For this review, take the finished solid that the model builds, in its own axes (mm). A direction names the side the tool comes from. Coordinates: 2 decimals unless noted, no trailing zeros. Write each loop counter-clockwise with the first axis right and the second up, starting at its lowest first coordinate (ties: lowest second). Pieces come first, ordered by that corner, then holes.
1) We need section A-A on x = 8.5. Write out the cut boundary in (y, z), then the cut area to 3 significant figures.
2) Insertion check: P1, Ø4, axis at y = 173, z = 5, coming from the -X side; P2, Ø20, axis at y = 129.5, z = 21, coming from the -X side; P3, Ø8, axis at x = -132.5, y = 162.5, coming from the -Z side. Each pin has a flat end and moves straight along its axis. Give the tip position at first contact, or say it passes through.
3) To check wall thickness, follow line 1 along X through (y, z) = (119, 62); line 2 along X through (y, z) = (77, -11); line 3 along Z through (x, y) = (95.5, 18). State the ranges of each line that lie inside material, in increasing order.
4) For faces 1 (the face through (30, 121, 35)), 2 (the face through (-30, 121, 35)), 3 (the face through (0.42, 150.516, 39.308)), 4 (the face through (225.952, 56.186, -8.941)), 5 (the face through (0.42, 91.14, 30.64)), list the 3-axis set-ups (+Z, -Z, +X, -X, +Y, -Y) from which the entire face can be reached by the end or side of a thin tool; tool diameter is ignored.
5) Mouldability with a two-part tool opening along X and no side actions: class faces 6 (the face through (-137.606, 96.84, -3.634)), 7 (the face through (-226.16, 56.69, -8.94)), 8 (the face through (-2, 0, -17)) as pulls with the +X half, pulls with the -X half, needs draft (parallel to the pull), parting line crosses it, or undercut.
from build123d import *

# Parameters (mm, degrees)
BOSS_EXTRUDE1_START     = -25
BOSS_EXTRUDE1_DEPTH     = 50
CUT_EXTRUDE1_DEPTH      = 341.53226913
CUT_EXTRUDE1_DEPTH_BACK = 341.53226913
BOSS_EXTRUDE3_DEPTH     = 30
CUT_EXTRUDE2_DEPTH      = 350.338594582
CUT_EXTRUDE2_DEPTH_BACK = 350.338594582
SKETCH4_R               = 20
CUT_EXTRUDE3_DEPTH      = 350.338594582
CUT_EXTRUDE3_DEPTH_BACK = 350.338594582
SKETCH6_R               = 12.5


# Read off the part's stored shape, not the designer's step: Boss-Extrude1
with BuildPart() as part:
    # Boss-Extrude1 outline → Boss-Extrude1 (new body)
    with BuildSketch(Plane.XY.offset(BOSS_EXTRUDE1_START)):
        with BuildLine():
            Line((175, 0), (215.218833807, 40.218833807))
            ThreePointArc((215.218833807, 40.218833807), (226.057471223, 56.440000887), (229.863494748, 75.574172084))
            add(Edge.make_bspline(
                [(229.863494748, 75.574172084), (229.863497015, 220.574172084), (130.657195822, 208), (130.657198498, 108), (160, 250), (60, 250)],
                knots=[0, 0, 0, 0, 0, 0, 1, 1, 1, 1, 1, 1], degree=5))
            Line((60, 250), (-60, 250))
            add(Edge.make_bspline(
                [(-60, 250), (-160, 250), (-130.657198498, 108), (-130.657195822, 208), (-229.863497015, 220.574172084), (-229.863494748, 75.574172084)],
                knots=[0, 0, 0, 0, 0, 0, 1, 1, 1, 1, 1, 1], degree=5))
            ThreePointArc((-229.863494748, 75.574172084), (-226.057471223, 56.440000887), (-215.218833807, 40.218833807))
            Line((-215.218833807, 40.218833807), (-175, 0))
            Line((-175, 0), (175, 0))
        make_face()
    extrude(amount=BOSS_EXTRUDE1_DEPTH)

    # Sketch2 → Cut-Extrude1 (cut, two sides: drawn at the far end of the back side and taken through both)
    with BuildSketch(Plane(origin=(0, 0, 0), x_dir=(0, 0, -1), z_dir=(1, 0, 0)).offset(-CUT_EXTRUDE1_DEPTH_BACK)):
        Polygon((23.039732542, -10), (-12.506441807, 260), (35, 260), (35, -10), align=None)
        Polygon((-23.039732542, 260), (12.506441807, -10), (-35, -10), (-35, 260), align=None)
    extrude(amount=CUT_EXTRUDE1_DEPTH + CUT_EXTRUDE1_DEPTH_BACK, mode=Mode.SUBTRACT)

    # Sketch11 → Boss-Extrude3 (add, symmetric)
    with BuildSketch(Plane(origin=(0, 0, 0), x_dir=(0, 0, -1), z_dir=(1, 0, 0))):
        Polygon((-9.148641973, 154.486691682), (-1.31707044, 95), (-60.803762122, 87.168428467), (-68.635333655, 146.655120149), align=None)
    extrude(amount=BOSS_EXTRUDE3_DEPTH, both=True)

    # Sketch4 → Cut-Extrude2 (cut, two sides: drawn at the far end of the back side and taken through both)
    with BuildSketch(Plane(origin=(0, 2.811189919, -21.353107392), x_dir=(-1, 0, 0), z_dir=(0, 0.13052619222005532, -0.99144486137381)).offset(-CUT_EXTRUDE2_DEPTH_BACK)):
        with Locations(Location((0, 124.321792579, 0), (0, 0, 90))):
            Circle(SKETCH4_R)
    extrude(amount=CUT_EXTRUDE2_DEPTH + CUT_EXTRUDE2_DEPTH_BACK, mode=Mode.SUBTRACT)

    # Sketch6 → Cut-Extrude3 (cut, two sides: drawn at the far end of the back side and taken through both)
    with BuildSketch(Plane(origin=(0, 2.811189919, -21.353107392), x_dir=(-1, 0, 0), z_dir=(0, 0.13052619222005532, -0.99144486137381)).offset(-CUT_EXTRUDE3_DEPTH_BACK)):
        with Locations(Location((150, 97.164552434, 0), (0, 0, 90))):
            Circle(SKETCH6_R)
    extrude(amount=CUT_EXTRUDE3_DEPTH + CUT_EXTRUDE3_DEPTH_BACK, mode=Mode.SUBTRACT)


solid = part.part
Result:
1. outline: (0, -21.72) - (108.12, -7.49) - (98.93, 62.35) - (87.17, 60.8) - (95, 1.32) - (0, -11.19) - close; (134.82, 67.08) - (144.02, -2.76) - (250, 11.19) - (250, 21.72) - (154.49, 9.15) - (146.66, 68.64) - close
1. area: 3,680 mm2
2. P1: stops at x = -197.25
2. P2: stops at x = -30
2. P3: stops at z = -0.86
3. line 1: x = -30 to -19.92, 19.92 to 30
3. line 2: x = -229.86 to 229.86
3. line 3: z = -19.35 to -8.82
4. face 1: +Z, +X, -Y
4. face 2: +Z, -X, -Y
4. face 3: +Z, +X, -X
4. face 4: +Z, -Z, +X, -Y
4. face 5: +X, -X, -Y
5. face 6: undercut
5. face 7: pulls with the -X half
5. face 8: needs draft
